The listing builds one solid part. Answer for the finished solid, in the listing's coordinates (mm). A direction names the side the tool comes from. Give positions to 0.01 mm unless a question says otherwise; leave off trailing zeros. Order: outer loops, then holes, each group sorted by start corner. A loop starts at its lowest first (then second) coordinate and runs counter-clockwise, first axis right, second up. Notation, with made-up numbers: (83, 22.25) - (111, 22.25) arc R19 ccw to (111, 49.25) - close; hole circle Ø7 at (-34.75, 23.5). An arc over 180 degrees is marked (long way). Answer in a Markdown table with one row per item. Add a question column.
```python
from build123d import *

# Parameters (mm, degrees)
EXTRUDE_1_DEPTH     = 7
SKETCH_2_R          = 15
EXTRUDE_2_DEPTH     = 18.4
EXTRUDE_3_DEPTH     = 7
EXTRUDE_START       = 6.3
SKETCH_4_R          = 15
EXTRUDE_4_DEPTH     = 6.3
SKETCH_5_R          = 15
EXTRUDE_5_DEPTH     = 6.3
CUT_EXTRUDE_1_DEPTH = 90.291681756


with BuildPart() as part:
    # 草图1 → 凸台-拉伸1 (new body)
    with BuildSketch(Plane.XY.offset(28.9)):
        with BuildLine():
            Line((42.411201909, 45.77806603), (42.129389286, 47.376304833))
            ThreePointArc((42.129389286, 47.376304833), (40.514502568, 47.409839327), (38.89961585, 47.376304833))
            Line((38.89961585, 47.376304833), (38.617803227, 45.77806603))
            ThreePointArc((38.617803227, 45.77806603), (37.528159676, 43.541003491), (35.420005537, 42.219088972))
            ThreePointArc((35.420005537, 42.219088972), (32.937471152, 42.04939837), (30.741018632, 43.218743572))
            Line((30.741018632, 43.218743572), (29.573606233, 44.346100621))
            ThreePointArc((29.573606233, 44.346100621), (28.247424353, 43.424024), (26.960664635, 42.447687427))
            Line((26.960664635, 42.447687427), (27.672094632, 40.98903977))
            ThreePointArc((27.672094632, 40.98903977), (28.10546685, 38.538741749), (27.176936184, 36.230148526))
            ThreePointArc((27.176936184, 36.230148526), (25.268265311, 34.633668845), (22.80397403, 34.288646587))
            Line((22.80397403, 34.288646587), (21.196873713, 34.514509808))
            ThreePointArc((21.196873713, 34.514509808), (20.665953073, 32.989024), (20.198818833, 31.442812735))
            Line((20.198818833, 31.442812735), (21.631749371, 30.680910052))
            ThreePointArc((21.631749371, 30.680910052), (23.422603901, 28.95330711), (24.028363863, 26.539839327))
            ThreePointArc((24.028363863, 26.539839327), (23.422603901, 24.126371544), (21.631749371, 22.398768602))
            Line((21.631749371, 22.398768602), (20.198818833, 21.63686592))
            ThreePointArc((20.198818833, 21.63686592), (20.665953073, 20.090654655), (21.196873713, 18.565168847))
            Line((21.196873713, 18.565168847), (22.80397403, 18.791032067))
            ThreePointArc((22.80397403, 18.791032067), (25.268265311, 18.446009809), (27.176936184, 16.849530129))
            ThreePointArc((27.176936184, 16.849530129), (28.10546685, 14.540936905), (27.672094632, 12.090638884))
            Line((27.672094632, 12.090638884), (26.960664635, 10.631991228))
            ThreePointArc((26.960664635, 10.631991228), (28.247424353, 9.655654655), (29.573606233, 8.733578033))
            Line((29.573606233, 8.733578033), (30.741018632, 9.860935083))
            ThreePointArc((30.741018632, 9.860935083), (32.937471152, 11.030280285), (35.420005536, 10.860589683))
            ThreePointArc((35.420005536, 10.860589683), (37.528159676, 9.538675164), (38.617803227, 7.301612625))
            Line((38.617803227, 7.301612625), (38.89961585, 5.703373822))
            ThreePointArc((38.89961585, 5.703373822), (40.514502568, 5.669839327), (42.129389286, 5.703373822))
            Line((42.129389286, 5.703373822), (42.411201909, 7.301612625))
            ThreePointArc((42.411201909, 7.301612625), (43.50084546, 9.538675164), (45.6089996, 10.860589683))
            ThreePointArc((45.6089996, 10.860589683), (48.091533984, 11.030280285), (50.287986504, 9.860935083))
            Line((50.287986504, 9.860935083), (51.455398903, 8.733578033))
            ThreePointArc((51.455398903, 8.733578033), (52.781580783, 9.655654655), (54.068340501, 10.631991228))
            Line((54.068340501, 10.631991228), (53.356910504, 12.090638884))
            ThreePointArc((53.356910504, 12.090638884), (52.923538286, 14.540936905), (53.852068952, 16.849530129))
            ThreePointArc((53.852068952, 16.849530129), (55.760739826, 18.446009809), (58.225031106, 18.791032067))
            Line((58.225031106, 18.791032067), (59.832131424, 18.565168847))
            ThreePointArc((59.832131424, 18.565168847), (60.363052063, 20.090654655), (60.830186304, 21.63686592))
            Line((60.830186304, 21.63686592), (59.397255765, 22.398768602))
            ThreePointArc((59.397255765, 22.398768602), (57.606401235, 24.126371544), (57.000641274, 26.539839327))
            ThreePointArc((57.000641274, 26.539839327), (57.606401235, 28.95330711), (59.397255765, 30.680910052))
            Line((59.397255765, 30.680910052), (60.830186304, 31.442812735))
            ThreePointArc((60.830186304, 31.442812735), (60.363052063, 32.989024), (59.832131424, 34.514509808))
            Line((59.832131424, 34.514509808), (58.225031106, 34.288646587))
            ThreePointArc((58.225031106, 34.288646587), (55.760739826, 34.633668845), (53.852068952, 36.230148526))
            ThreePointArc((53.852068952, 36.230148526), (52.923538286, 38.538741749), (53.356910504, 40.98903977))
            Line((53.356910504, 40.98903977), (54.068340501, 42.447687427))
            ThreePointArc((54.068340501, 42.447687427), (52.781580783, 43.424024), (51.455398903, 44.346100621))
            Line((51.455398903, 44.346100621), (50.287986504, 43.218743572))
            ThreePointArc((50.287986504, 43.218743572), (48.091533984, 42.04939837), (45.6089996, 42.219088972))
            ThreePointArc((45.6089996, 42.219088972), (43.50084546, 43.541003491), (42.411201909, 45.77806603))
        make_face()
    extrude(amount=-EXTRUDE_1_DEPTH)

    # 草图2 → 凸台-拉伸2 (add)
    with BuildSketch(Plane(origin=(0, 0, 21.9), x_dir=(-1, 0, 0), z_dir=(0, 0, -1))):
        with Locations((-40.514502568, 26.539839327)):
            Circle(SKETCH_2_R)
    extrude(amount=EXTRUDE_2_DEPTH)

    # 草图3 → 凸台-拉伸3 (add)
    with BuildSketch(Plane.XY.offset(3.5)):
        with BuildLine():
            Line((42.411201909, 45.77806603), (42.129389286, 47.376304833))
            ThreePointArc((42.129389286, 47.376304833), (40.514502568, 47.409839327), (38.89961585, 47.376304833))
            Line((38.89961585, 47.376304833), (38.617803227, 45.77806603))
            ThreePointArc((38.617803227, 45.77806603), (37.528159676, 43.541003491), (35.420005537, 42.219088972))
            ThreePointArc((35.420005537, 42.219088972), (32.937471152, 42.04939837), (30.741018632, 43.218743572))
            Line((30.741018632, 43.218743572), (29.573606233, 44.346100621))
            ThreePointArc((29.573606233, 44.346100621), (28.247424353, 43.424024), (26.960664635, 42.447687427))
            Line((26.960664635, 42.447687427), (27.672094632, 40.98903977))
            ThreePointArc((27.672094632, 40.98903977), (28.10546685, 38.538741749), (27.176936184, 36.230148526))
            ThreePointArc((27.176936184, 36.230148526), (25.268265311, 34.633668845), (22.80397403, 34.288646587))
            Line((22.80397403, 34.288646587), (21.196873713, 34.514509808))
            ThreePointArc((21.196873713, 34.514509808), (20.665953073, 32.989024), (20.198818833, 31.442812735))
            Line((20.198818833, 31.442812735), (21.631749371, 30.680910052))
            ThreePointArc((21.631749371, 30.680910052), (23.422603901, 28.95330711), (24.028363863, 26.539839327))
            ThreePointArc((24.028363863, 26.539839327), (23.422603901, 24.126371544), (21.631749371, 22.398768602))
            Line((21.631749371, 22.398768602), (20.198818833, 21.63686592))
            ThreePointArc((20.198818833, 21.63686592), (20.665953073, 20.090654655), (21.196873713, 18.565168847))
            Line((21.196873713, 18.565168847), (22.80397403, 18.791032067))
            ThreePointArc((22.80397403, 18.791032067), (25.268265311, 18.446009809), (27.176936184, 16.849530129))
            ThreePointArc((27.176936184, 16.849530129), (28.10546685, 14.540936905), (27.672094632, 12.090638884))
            Line((27.672094632, 12.090638884), (26.960664635, 10.631991228))
            ThreePointArc((26.960664635, 10.631991228), (28.247424353, 9.655654655), (29.573606233, 8.733578033))
            Line((29.573606233, 8.733578033), (30.741018632, 9.860935083))
            ThreePointArc((30.741018632, 9.860935083), (32.937471152, 11.030280285), (35.420005536, 10.860589683))
            ThreePointArc((35.420005536, 10.860589683), (37.528159676, 9.538675164), (38.617803227, 7.301612625))
            Line((38.617803227, 7.301612625), (38.89961585, 5.703373822))
            ThreePointArc((38.89961585, 5.703373822), (40.514502568, 5.669839327), (42.129389286, 5.703373822))
            Line((42.129389286, 5.703373822), (42.411201909, 7.301612625))
            ThreePointArc((42.411201909, 7.301612625), (43.50084546, 9.538675164), (45.6089996, 10.860589683))
            ThreePointArc((45.6089996, 10.860589683), (48.091533984, 11.030280285), (50.287986504, 9.860935083))
            Line((50.287986504, 9.860935083), (51.455398903, 8.733578033))
            ThreePointArc((51.455398903, 8.733578033), (52.781580783, 9.655654655), (54.068340501, 10.631991228))
            Line((54.068340501, 10.631991228), (53.356910504, 12.090638884))
            ThreePointArc((53.356910504, 12.090638884), (52.923538286, 14.540936905), (53.852068952, 16.849530129))
            ThreePointArc((53.852068952, 16.849530129), (55.760739826, 18.446009809), (58.225031106, 18.791032067))
            Line((58.225031106, 18.791032067), (59.832131424, 18.565168847))
            ThreePointArc((59.832131424, 18.565168847), (60.363052063, 20.090654655), (60.830186304, 21.63686592))
            Line((60.830186304, 21.63686592), (59.397255765, 22.398768602))
            ThreePointArc((59.397255765, 22.398768602), (57.606401235, 24.126371544), (57.000641274, 26.539839327))
            ThreePointArc((57.000641274, 26.539839327), (57.606401235, 28.95330711), (59.397255765, 30.680910052))
            Line((59.397255765, 30.680910052), (60.830186304, 31.442812735))
            ThreePointArc((60.830186304, 31.442812735), (60.363052063, 32.989024), (59.832131424, 34.514509808))
            Line((59.832131424, 34.514509808), (58.225031106, 34.288646587))
            ThreePointArc((58.225031106, 34.288646587), (55.760739826, 34.633668845), (53.852068952, 36.230148526))
            ThreePointArc((53.852068952, 36.230148526), (52.923538286, 38.538741749), (53.356910504, 40.98903977))
            Line((53.356910504, 40.98903977), (54.068340501, 42.447687427))
            ThreePointArc((54.068340501, 42.447687427), (52.781580783, 43.424024), (51.455398903, 44.346100621))
            Line((51.455398903, 44.346100621), (50.287986504, 43.218743572))
            ThreePointArc((50.287986504, 43.218743572), (48.091533984, 42.04939837), (45.6089996, 42.219088972))
            ThreePointArc((45.6089996, 42.219088972), (43.50084546, 43.541003491), (42.411201909, 45.77806603))
        make_face()
    extrude(amount=-EXTRUDE_3_DEPTH)

    # 草图4 → 凸台-拉伸4 (add)
    with BuildSketch(Plane.XY.offset(28.9).offset(EXTRUDE_START)):
        with Locations(Location((40.514502568, 26.539839327, 0), (0, 0, 180))):
            Circle(SKETCH_4_R)
    extrude(amount=-EXTRUDE_4_DEPTH)

    # 草图5 → 凸台-拉伸5 (add)
    with BuildSketch(Plane(origin=(0, 0, -3.5), x_dir=(-1, 0, 0), z_dir=(0, 0, -1))):
        with Locations((-40.514502568, 26.539839327)):
            Circle(SKETCH_5_R)
    extrude(amount=EXTRUDE_5_DEPTH)

    # 草图6 → 切除-拉伸1 (cut, through all)
    with BuildSketch(Plane(origin=(0, 0, -9.8), x_dir=(-1, 0, 0), z_dir=(0, 0, -1))):
        with BuildLine():
            Line((-38.971830845, 31.295905344), (-38.971830845, 34.262802089))
            Line((-38.971830845, 34.262802089), (-41.953176795, 34.262802089))
            Line((-41.953176795, 34.262802089), (-41.953176795, 31.328389888))
            ThreePointArc((-41.953176795, 31.328389888), (-40.568978996, 21.540136104), (-38.971830845, 31.295905344))
        make_face()
    extrude(amount=-CUT_EXTRUDE_1_DEPTH, mode=Mode.SUBTRACT)


solid = part.part
```
(1) Find section D-D, the plane y = 20.5. Write down the section's boundary in (x, z), plus the area to 3 significant figures.
(2) Each of these flat-tipped pins is pushed along its axis until it touches: P1, Ø0.9, axis at x = 40.5, z = 19.5, coming from the -Y side; P2, Ø1.5, axis at x = 44.5, z = 9, coming from the +Y side; P3, Ø13, axis at x = 40.51, y = 26.54, coming from the -Z side; P4, Ø6, axis at y = 38, z = 18, coming from the -X side. Where does it stop, or does it pass through?
(3) Straight lines are drawn through the part: line 1 (Z direction, x = 32, y = 42); line 2 (Y direction, x = 40, z = 23.5); line 3 (Y direction, x = 34, z = 24). For each, find the intervals that lie inside material, in ascending order.
(4) Find section A-A, the plane y = 32.5. Write down the section's boundary in (x, z), plus the area to 3 significant figures.
(5) Find section C-C, the plane x = 37.5. Write down the section's boundary in (y, z).
(6) The mould has two halves that part along Y. Classify faces 4 (the face through (42.27, 6.49, 0.05)), 5 (the face through (23.44, 24.16, 0.05)), 6 (the face through (37.552, 43.567, 0.049)): +Y half, -Y half, draft (parallel to the pull), parting line (faces both ways), or undercut.
(7) For faces 1 (the face through (37.552, 43.567, 25.449)), 2 (the face through (59.02, 18.68, 0.05)), 3 (the face through (60, 31, 25)), determine the directions among +Z, -Z, +X, -X, +Y, -Y from which every point of the face is accessible in a straight line to the end or side of a thin tool.
(8) Find section B-B, the plane z = 5.5. Write down the section's boundary in (x, y).
Answer key:
| question | item | result |
|---|---|---|
| 1 | outline | (20.54, -3.5) - (26.78, -3.5) - (26.78, -9.8) - (54.24, -9.8) - (54.24, -3.5) - (60.49, -3.5) - (60.49, 3.5) - (54.24, 3.5) - (54.24, 21.9) - (60.49, 21.9) - (60.49, 28.9) - (54.24, 28.9) - (54.24, 35.2) - (26.78, 35.2) - (26.78, 28.9) - (20.54, 28.9) - (20.54, 21.9) - (26.78, 21.9) - (26.78, 3.5) - (20.54, 3.5) - close |
| 1 | area | 1,410 mm² |
| 2 | P1 | y = 11.54 |
| 2 | P2 | y = 41.19 |
| 2 | P3 | z = -9.8 |
| 2 | P4 | x = 28.13 |
| 3 | line 1 | -3.5 to 3.5, 21.9 to 28.9 |
| 3 | line 2 | 5.67 to 21.57, 34.26 to 47.41 |
| 3 | line 3 | 11.13 to 41.95 |
| 4 | outline | (20.51, -3.5) - (26.75, -3.5) - (26.75, -9.8) - (38.97, -9.8) - (38.97, 35.2) - (26.75, 35.2) - (26.75, 28.9) - (20.51, 28.9) - (20.51, 21.9) - (26.75, 21.9) - (26.75, 3.5) - (20.51, 3.5) - close; (41.95, -9.8) - (54.28, -9.8) - (54.28, -3.5) - (60.52, -3.5) - (60.52, 3.5) - (54.28, 3.5) - (54.28, 21.9) - (60.52, 21.9) - (60.52, 28.9) - (54.28, 28.9) - (54.28, 35.2) - (41.95, 35.2) - close |
| 4 | area | 1,280 mm² |
| 5 | outline | (9.57, -3.5) - (11.85, -3.5) - (11.85, -9.8) - (22.55, -9.8) - (22.55, 35.2) - (11.85, 35.2) - (11.85, 28.9) - (9.57, 28.9) - (9.57, 21.9) - (11.85, 21.9) - (11.85, 3.5) - (9.57, 3.5) - close; (30.53, -9.8) - (41.23, -9.8) - (41.23, -3.5) - (43.51, -3.5) - (43.51, 3.5) - (41.23, 3.5) - (41.23, 21.9) - (43.51, 21.9) - (43.51, 28.9) - (41.23, 28.9) - (41.23, 35.2) - (30.53, 35.2) - close |
| 6 | face 4 | -Y half |
| 6 | face 5 | undercut |
| 6 | face 6 | +Y half |
| 7 | face 1 | +Z, -Z, +Y |
| 7 | face 2 | +Z, -Z, -Y |
| 7 | face 3 | +Z, -Z, +X |
| 8 | outline | circle Ø30 at (40.51, 26.54); hole (38.97, 31.3) arc R5 ccw (long way) to (41.95, 31.33) - (41.95, 34.26) - (38.97, 34.26) - close |
